from build123d import *

# Parameters (mm, degrees)
SKETCH1_W           = 172.974
SKETCH1_H           = 102.108
BOSS_EXTRUDE1_DEPTH = 13.97
SKETCH2_R           = 7.4676
SKETCH2_R_2         = 3.014975044
SKETCH2_W           = 7.81218406
SKETCH2_H           = 2.407827673
BOSS_EXTRUDE3_DEPTH = 3.048
SKETCH3_R           = 7.4676
SKETCH3_R_2         = 3.014975044
BOSS_EXTRUDE5_DEPTH = 3.048
SKETCH4_R           = 3.175
CUT_EXTRUDE1_DEPTH  = 11.176


with BuildPart() as part:
    # Sketch1 → Boss-Extrude1 (new body)
    with BuildSketch(Plane.XY):
        with Locations((58.9637029, 33.169946412)):
            Rectangle(SKETCH1_W, SKETCH1_H)
        with BuildLine():
            Line((-27.5232971, 84.223946412), (-43.0172971, 84.223946412))
            ThreePointArc((-43.0172971, 84.223946412), (-57.385706894, 78.272356205), (-63.3372971, 63.903946412))
            Line((-63.3372971, 63.903946412), (-63.3372971, 2.435946412))
            ThreePointArc((-63.3372971, 2.435946412), (-57.385706894, -11.932463382), (-43.0172971, -17.884053588))
            Line((-43.0172971, -17.884053588), (-27.5232971, -17.884053588))
            Line((-27.5232971, -17.884053588), (-27.5232971, 84.223946412))
        make_face()
        with BuildLine():
            Line((160.9447029, 84.223946412), (145.4507029, 84.223946412))
            Line((145.4507029, 84.223946412), (145.4507029, -17.884053588))
            Line((145.4507029, -17.884053588), (160.9447029, -17.884053588))
            ThreePointArc((160.9447029, -17.884053588), (175.313112694, -11.932463382), (181.2647029, 2.435946412))
            Line((181.2647029, 2.435946412), (181.2647029, 63.903946412))
            ThreePointArc((181.2647029, 63.903946412), (175.313112694, 78.272356205), (160.9447029, 84.223946412))
        make_face()
    extrude(amount=BOSS_EXTRUDE1_DEPTH)

    # Sketch2 → Boss-Extrude3 (add)
    with BuildSketch(Plane(origin=(0, 0, 0), x_dir=(-1, 0, 0), z_dir=(0, 0, -1))):
        with Locations(Location((-163.4847029, 58.823946412, 0), (0, 0, 180))):
            Circle(SKETCH2_R)
        with Locations(Location((-170.337090886, 26.676001086, 0), (0, 0, 180))):
            Circle(SKETCH2_R_2)
        with Locations(Location((-163.221177768, 32.823656386, 0), (0, 0, 180))):
            Circle(SKETCH2_R_2)
        with Locations(Location((-156.732358191, 26.205188985, 0), (0, 0, 180))):
            Circle(SKETCH2_R_2)
        with Locations(Location((-163.721455714, 19.973644896, 0), (0, 0, 180))):
            Circle(SKETCH2_R_2)
        with Locations((-152.730393721, 74.856056835)):
            Rectangle(SKETCH2_W, SKETCH2_H)
    extrude(amount=BOSS_EXTRUDE3_DEPTH)

    # Sketch3 → Boss-Extrude5 (add)
    with BuildSketch(Plane(origin=(0, 0, 0), x_dir=(-1, 0, 0), z_dir=(0, 0, -1))):
        with Locations(Location((45.487523866, 28.516423037, 0), (0, 0, 180))):
            Circle(SKETCH3_R)
        with Locations(Location((44.957454366, 53.116068624, 0), (0, 0, 180))):
            Circle(SKETCH3_R_2)
        with Locations(Location((38.341819194, 59.818424813, 0), (0, 0, 180))):
            Circle(SKETCH3_R_2)
        with Locations(Location((45.457732312, 65.966080113, 0), (0, 0, 180))):
            Circle(SKETCH3_R_2)
        with Locations(Location((51.94655189, 59.347612713, 0), (0, 0, 180))):
            Circle(SKETCH3_R_2)
        Polygon((38.47340824, 76.391412748), (41.190295926, 76.391412748), (41.190295926, 73.983585075), (38.47340824, 73.983585075), (38.47340824, 71.443585075), (35.93340824, 71.443585075), (35.93340824, 73.983585075), (33.570295926, 73.983585075), (33.570295926, 76.391412748), (35.93340824, 76.391412748), (35.93340824, 78.931412748), (38.47340824, 78.931412748), align=None)
    extrude(amount=BOSS_EXTRUDE5_DEPTH)

    # Sketch4 → Cut-Extrude1 (cut)
    with BuildSketch(Plane(origin=(0, 84.223946412, 0), x_dir=(1, 0, 0), z_dir=(0, 1, 0))):
        with Locations(Location((-12.641077469, -7.400069152, 0), (0, 0, 270))):
            Circle(SKETCH4_R)
    extrude(amount=-CUT_EXTRUDE1_DEPTH, mode=Mode.SUBTRACT)


solid = part.part
Design review of the part built by this model. Coordinates are the model's own, in mm. A direction names the side the tool comes from. Coordinates: 2 decimals unless noted, no trailing zeros. Order: outer loops, then holes, each group sorted by start corner. A loop starts at its lowest first (then second) coordinate and runs counter-clockwise, first axis right, second up.
Item 1: Take a section at B-B, the plane x = 39. Write out the cut boundary in (y, z).
Item 2: For pin 1 Ø8 at (y, z) = (50.5, -1) entering from -X; pin 2 Ø1.9 at (y, z) = (74.5, -1) entering from -X; pin 3 Ø1.3 at (y, z) = (77.5, -1) entering from +X; pin 4 Ø2 at (y, z) = (78, -2) entering from -X, all flat-tipped, find the tip position at first contact; note any pin that passes through.
Item 3: The part is to be moulded in two halves that separate along X. For faces 1 (the cylindrical face through (-43.34, 50.57, -1.5)), 2 (the cylindrical face through (175.47, 78.114, 6.887)), 3 (the flat face through (-63.337, 34, 7)), say which applies: pulls with the +X half, pulls with the -X half, needs draft (parallel to the pull), parting line crosses it, or undercut.
Item 4: For line 1 (X direction, y = 76, z = -1.5); line 2 (Z direction, x = 103, y = -3.5); line 3 (X direction, y = 78.5, z = -2), list the stretches that pass through material, from the lowest coordinate up.
Item 5: Take a section at C-C, the plane y = 9. Write out the cut boundary in (x, z), then the cut area to 3 significant figures.
Item 6: Take a section at A-A, the plane z = 8. Write out the cut boundary in (x, y).
Item 7: For faces 4 (the flat face through (157, 26, -3.048)), 5 (the cylindrical face through (-15.74, 78.71, 6.71)), 6 (the cylindrical face through (159.5, 27.4, -1.5)), list the 3-axis set-ups (+Z, -Z, +X, -X, +Y, -Y) from which the entire face can be reached by the end or side of a thin tool; tool diameter is ignored.
The answers:
1. outline: (-17.88, 0) - (84.22, 0) - (84.22, 13.97) - (-17.88, 13.97) - close
2. pin 1: stops at x = -63.34
2. pin 2: stops at x = -41.19
2. pin 3: stops at x = -35.93
2. pin 4: stops at x = -38.47
3. face 1: undercut
3. face 2: pulls with the +X half
3. face 3: pulls with the -X half
4. line 1: x = -41.19 to -33.57, 148.82 to 156.64
4. line 2: z = 0 to 13.97
4. line 3: x = -38.47 to -35.93
5. outline: (-63.34, 0) - (181.26, 0) - (181.26, 13.97) - (-63.34, 13.97) - close
5. area: 3,420 mm2
6. outline: (-63.34, 2.44) arc R20.32 ccw to (-43.02, -17.88) - (160.94, -17.88) arc R20.32 ccw to (181.26, 2.44) - (181.26, 63.9) arc R20.32 ccw to (160.94, 84.22) - (-9.52, 84.22) - (-9.52, 73.05) - (-15.76, 73.05) - (-15.76, 84.22) - (-43.02, 84.22) arc R20.32 ccw to (-63.34, 63.9) - close
7. face 4: -Z, +X, -X, +Y, -Y
7. face 5: +Y
7. face 6: -Z
